Here's how the part is built. I have some questions about the finished solid (model axes, mm). Round coordinates to 2 decimals unless told otherwise and drop trailing zeros. Write each loop counter-clockwise with the first axis right and the second up, starting at its lowest first coordinate (ties: lowest second). Pieces come first, ordered by that corner, then holes. Notation, with made-up numbers: (0, 39) -> (16, 39) arc R7 cw to (16, 47) -> close; hole circle Ø7 at (88, 48). An arc over 180 degrees is marked (long way). Answer in a Markdown table with one row per item. Add a question column.
from build123d import *

# Parameters (mm, degrees)
SKETCH1_W               = 25
SKETCH1_H               = 150
BOSS_EXTRUDE1_DEPTH     = 0.4
SKETCH2_R               = 1.38
CUT_EXTRUDE1_DEPTH      = 0.4
MIRROR2_COPY_1_SKETCH_R = 1.38
MIRROR2_COPY_1_DEPTH    = 0.4


with BuildPart() as part:
    # Sketch1 → Boss-Extrude1 (new body)
    with BuildSketch(Plane(origin=(0, 0, 0), x_dir=(1, 0, 0), z_dir=(0, 1, 0))):
        Rectangle(SKETCH1_W, SKETCH1_H)
    extrude(amount=BOSS_EXTRUDE1_DEPTH)

    # Sketch2 → Cut-Extrude1 (cut)
    with BuildSketch(Plane(origin=(0, 0.4, 0), x_dir=(1, 0, 0), z_dir=(0, 1, 0))):
        with Locations((-10, 66)):
            Circle(SKETCH2_R)
    cut_extrude1 = extrude(amount=-CUT_EXTRUDE1_DEPTH, mode=Mode.SUBTRACT)

    # Mirror1: Cut-Extrude1 across plane
    add(cut_extrude1.mirror(Plane(origin=(0, 0, 0), x_dir=(0, 0, 1), z_dir=(1, 0, 0))), mode=Mode.SUBTRACT)

    # Mirror2: Cut-Extrude1 across plane
    add(cut_extrude1.mirror(Plane.XY), mode=Mode.SUBTRACT)

    # Mirror2 copy 1 sketch → Mirror2 copy 1 (cut)
    with BuildSketch(Plane(origin=(0, 0.4, 0), x_dir=(-1, 0, 0), z_dir=(0, 1, 0))):
        with Locations((-10, 66)):
            Circle(MIRROR2_COPY_1_SKETCH_R)
    extrude(amount=-MIRROR2_COPY_1_DEPTH, mode=Mode.SUBTRACT)


solid = part.part
Item 1: If we section it at B-B on x = 10: Please give me the cut outline in (y, z), then the cut area to 3 significant figures.
Item 2: I need wall thicknesses on line 1 along X through (y, z) = (0.2, -66); line 2 along Z through (x, y) = (10, 0.15); line 3 along X through (y, z) = (0.3, -67). Which ranges of each line are inside material? Lowest first, please. Write a range as from..to.
Item 3: If we mould it in two halves opening along X, with no side actions, what happens to faces 1 (the flat face through (0, 0.4, -1)), 2 (the cylindrical face through (-9.258, 0.203, 67.164))? For each: pulls with the +X half, pulls with the -X half, needs draft (parallel to the pull), parting line crosses it, or undercut.
Item 4: If we section it at A-A on z = -66: Please give me the cut outline in (x, y).
Results list:
| question | item | result |
|---|---|---|
| 1 | outline | (0, -75) -> (0.4, -75) -> (0.4, -67.38) -> (0, -67.38) -> close; (0, -64.62) -> (0.4, -64.62) -> (0.4, 64.62) -> (0, 64.62) -> close; (0, 67.38) -> (0.4, 67.38) -> (0.4, 75) -> (0, 75) -> close |
| 1 | area | 57.8 mm² |
| 2 | line 1 | -12.5..-11.38, -8.62..8.62, 11.38..12.5 |
| 2 | line 2 | -75..-67.38, -64.62..64.62, 67.38..75 |
| 2 | line 3 | -12.5..-10.95, -9.05..9.05, 10.95..12.5 |
| 3 | face 1 | needs draft |
| 3 | face 2 | undercut |
| 4 | outline | (-12.5, 0) -> (-11.38, 0) -> (-11.38, 0.4) -> (-12.5, 0.4) -> close; (-8.62, 0) -> (8.62, 0) -> (8.62, 0.4) -> (-8.62, 0.4) -> close; (11.38, 0) -> (12.5, 0) -> (12.5, 0.4) -> (11.38, 0.4) -> close |
